Geometry check sheet. Reference: the model listing, model coordinates, mm. Face numbers are marked on the shaded views. A direction names the side the tool comes from. Give positions to 0.01 mm unless a question says otherwise; leave off trailing zeros. Write each loop counter-clockwise with the first axis right and the second up, starting at its lowest first coordinate (ties: lowest second). Pieces come first, ordered by that corner, then holes. Notation, with made-up numbers: (-24.75, 57.5) - (-11.75, 57.5) arc R27 cw to (-11.75, 92.5) - close; hole circle Ø4 at (61, -2). An arc over 180 degrees is marked (long way). Write item = value, one per line. Start each with the question number.
(1) Draft check along Y on the marked faces 1, 2 and 3. Enter one of: pulls with the +Y half, pulls with the -Y half, needs draft (parallel to the pull), parting line crosses it, or undercut.
(2) Access from +Z, -Z, +X, -X, +Y, -Y to the whole of each face (thin tool, end or side, straight path). Record for the marked faces 4, 5 and 6.
(3) Thickness scan on L1, parallel to Z at x = 13.5, y = -5; L2, parallel to Z at x = -17, y = 22.5; L3, parallel to X at y = -27, z = -43.5. Record the ranges inside material, lowest first.
(4) Section check A-A, the plane z = 0. Enter the section's corners in (x, y) (3 decimals), plus the area to 3 significant figures.
(5) Section check C-C, the plane x = 4. Enter the section's corners in (y, z) (3 decimals).
(6) Section check B-B, the plane x = 17.5. Enter the section's corners in (y, z) (3 decimals), plus the area to 3 significant figures.
(7) Depth check by flat-ended pin: pin 1 Ø2 at (x, z) = (-1, 23) entering from +Y; pin 2 Ø1 at (x, z) = (-9, -43.5) entering from +Y; pin 3 Ø19 at (y, z) = (0, 0) entering from -X; pin 4 Ø5 at (x, z) = (-23.5, 29.5) entering from +Y. Enter the tip coordinate at first touch or a pass-through.
```python
from build123d import *

# Parameters (mm, degrees)
SKETCH2_R          = 15.875
CUT_EXTRUDE1_DEPTH = 64.5
FILLET2_R          = 10.16
FILLET3_R          = 10.16


with BuildPart() as part:
    # Sketch1 → Revolve2 (revolve)
    with BuildSketch(Plane.XY):
        Polygon((-31.75, -0.729526652), (-31.75, 24.670473348), (-12.7, 24.670473348), (-12.7, 75.470473348), (-31.75, 75.470473348), (-31.75, 100.870473348), (31.75, 100.870473348), (31.75, 75.470473348), (12.7, 75.470473348), (12.7, 24.670473348), (31.75, 24.670473348), (31.75, -0.729526652), align=None)
    revolve(axis=Axis((-31.75, -0.729526652, 0), (1, 0, 0)))

    # Sketch2 → Cut-Extrude1 (cut, through all)
    with BuildSketch(Plane(origin=(31.75, 0, 0), x_dir=(0, 0, -1), z_dir=(1, 0, 0))):
        Circle(SKETCH2_R)
    extrude(amount=-CUT_EXTRUDE1_DEPTH, mode=Mode.SUBTRACT)

    # Fillet2
    fillet2_edges = [part.edges().sort_by_distance(p)[0] for p in [
        (31.75, -102.329526652, 0),
    ]]
    fillet(fillet2_edges, radius=FILLET2_R)

    # Fillet3
    fillet3_edges = [part.edges().sort_by_distance(p)[0] for p in [
        (-31.75, -102.329526652, 0),
    ]]
    fillet(fillet3_edges, radius=FILLET3_R)


solid = part.part
```
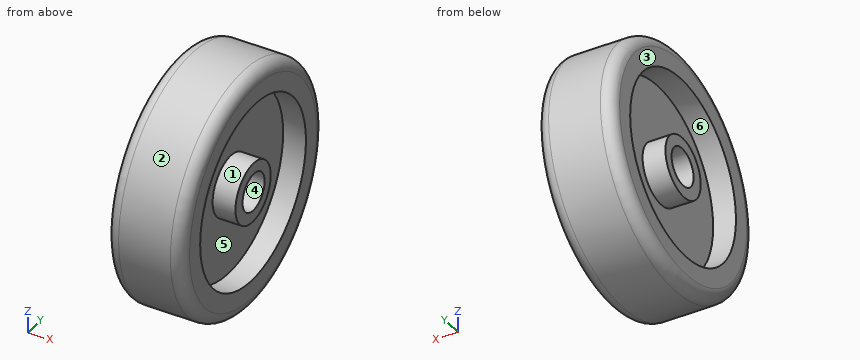
Model answer:
q1.face_1 = undercut
q1.face_2 = parting line crosses it
q1.face_3 = needs draft
q2.face_4 = +X, -X
q2.face_5 = +X
q2.face_6 = -X
q3.L1 = -101.51 to -76.08, -25.04 to -15.07, 15.07 to 25.04, 76.08 to 101.51
q3.L2 = -98.91 to -72.57, -10.27 to 10.27, 72.57 to 98.91
q3.L3 = -12.7 to 12.7
q4.outline = (-31.75, -92.17) arc R10.16 ccw to (-21.59, -102.33) - (21.59, -102.33) arc R10.16 ccw to (31.75, -92.17) - (31.75, -76.93) - (12.7, -76.93) - (12.7, -26.13) - (31.75, -26.13) - (31.75, -15.875) - (-31.75, -15.875) - (-31.75, -26.13) - (-12.7, -26.13) - (-12.7, -76.93) - (-31.75, -76.93) - close; (-31.75, 15.875) - (31.75, 15.875) - (31.75, 24.67) - (12.7, 24.67) - (12.7, 75.47) - (31.75, 75.47) - (31.75, 90.71) arc R10.16 ccw to (21.59, 100.87) - (-21.59, 100.87) arc R10.16 ccw to (-31.75, 90.71) - (-31.75, 75.47) - (-12.7, 75.47) - (-12.7, 24.67) - (-31.75, 24.67) - close
q4.area = 6,930 mm²
q5.outline = circle Ø203.2 at (-0.73, 0); hole circle Ø31.75 at (0, 0)
q6.outline = circle Ø203.2 at (-0.73, 0); circle Ø50.8 at (-0.73, 0); hole circle Ø152.4 at (-0.73, 0); hole circle Ø31.75 at (0, 0)
q6.area = 15,400 mm²
q7.pin_1 = 98.46
q7.pin_2 = 91.32
q7.pin_3 = through
q7.pin_4 = 97.12
